```python
from build123d import *

# Parameters (mm, degrees)
F0_R            = 87.5
F0_R_2          = 57.5
F1_DEPTH        = 5
F2_R            = 5
F3_DEPTH        = 5.001
F3_COPIES_COUNT = 6


# Not quite as in the source:
# - a pattern or mirror of a feature is missing from the dataset's text; its kind, count and spacing are read off the source's solid


with BuildPart() as f1:
    # F0 (on Front) → F1 (new body)
    with BuildSketch(Plane.XZ):
        Circle(F0_R)
        Circle(F0_R_2, mode=Mode.SUBTRACT)
    extrude(amount=F1_DEPTH)

    # F2 (on face) → F3 (cut, through all)
    with BuildSketch(Plane.XZ.offset(5)):
        with Locations((0, 72.5)):
            Circle(F2_R)
    f3 = extrude(amount=-F3_DEPTH, mode=Mode.SUBTRACT)

    # F3_copies: F3 ×6 about axis
    f3_copies_axis = Axis((0, 0, 0), (0, 1, 0))
    for i in range(1, F3_COPIES_COUNT):
        add(f3.rotate(f3_copies_axis, i * 360 / F3_COPIES_COUNT), mode=Mode.SUBTRACT)


solid = f1.part
```
The listing builds one solid part. Answer for the finished solid, in the listing's coordinates (mm). Give positions to 0.01 mm unless a question says otherwise; leave off trailing zeros. Write each loop counter-clockwise with the first axis right and the second up, starting at its lowest first coordinate (ties: lowest second). Pieces come first, ordered by that corner, then holes. Notation, with made-up numbers: (32.25, -12.5) - (74.25, -12.5) arc R27 ccw to (74.25, 21.5) - close; hole circle Ø1 at (-15, 74). An arc over 180 degrees is marked (long way). Use one line per item in the form item = value. Start each with the question number.
1) Find section D-D on y = -0.95. Determine the outline of the cut face in (x, z).
2) Find section C-C on x = 42. Determine the outline of the cut face in (y, z).
3) The mould has two halves that part along Z. Classify faces 1 (the face through (-12.465, -2.465, -56.133)), 2 (the face through (57, -5, 21)), 3 (the face through (-64.49, -2.46, 59.14)): pulls with the +Z half, pulls with the -Z half, needs draft (parallel to the pull), parting line crosses it, or undercut.
4) Find section A-A on x = 0. Determine the outline of the cut face in (y, z), plus the area to 3 significant figures.
5) Consider line 1 along Z through (x, y) = (0, -1.9); line 2 along X through (y, z) = (-3.8, -35); line 3 along X through (y, z) = (-1.2, -33.5). Determine where each line is inside the solid, lowest interval first. Write a range as from..to.
6) Flat-ended cylindrical pins translate along their axes: pin 1 Ø2 at (y, z) = (-3.5, -59) entering from -X; pin 2 Ø3 at (x, y) = (7, -1.5) entering from -Z; pin 3 Ø2 at (x, y) = (46.5, -1.5) entering from -Z. Find the tip coordinate at first contact, or state that the pin passes through.
7) Find section B-B on z = 0. Determine the outline of the cut face in (x, y).
Geometry results:
q1.outline = circle Ø175 at (0, 0); hole circle Ø10 at (-62.79, -36.25); hole circle Ø10 at (-62.79, 36.25); hole circle Ø115 at (0, 0); hole circle Ø10 at (0, -72.5); hole circle Ø10 at (0, 72.5); hole circle Ø10 at (62.79, -36.25); hole circle Ø10 at (62.79, 36.25)
q2.outline = (-5, -76.76) - (0, -76.76) - (0, -39.27) - (-5, -39.27) - close; (-5, 39.27) - (0, 39.27) - (0, 76.76) - (-5, 76.76) - close
q3.face_1 = undercut
q3.face_2 = needs draft
q3.face_3 = parting line crosses it
q4.outline = (-5, -87.5) - (0, -87.5) - (0, -77.5) - (-5, -77.5) - close; (-5, -67.5) - (0, -67.5) - (0, -57.5) - (-5, -57.5) - close; (-5, 57.5) - (0, 57.5) - (0, 67.5) - (-5, 67.5) - close; (-5, 77.5) - (0, 77.5) - (0, 87.5) - (-5, 87.5) - close
q4.area = 200 mm2
q5.line_1 = -87.5..-77.5, -67.5..-57.5, 57.5..67.5, 77.5..87.5
q5.line_2 = -80.2..-67.63, -57.95..-45.62, 45.62..57.95, 67.63..80.2
q5.line_3 = -80.83..-66.96, -58.61..-46.73, 46.73..58.61, 66.96..80.83
q6.pin_1 = -65.52
q6.pin_2 = -87.33
q6.pin_3 = -74.74
q7.outline = (-87.5, -5) - (-57.5, -5) - (-57.5, 0) - (-87.5, 0) - close; (57.5, -5) - (87.5, -5) - (87.5, 0) - (57.5, 0) - close
